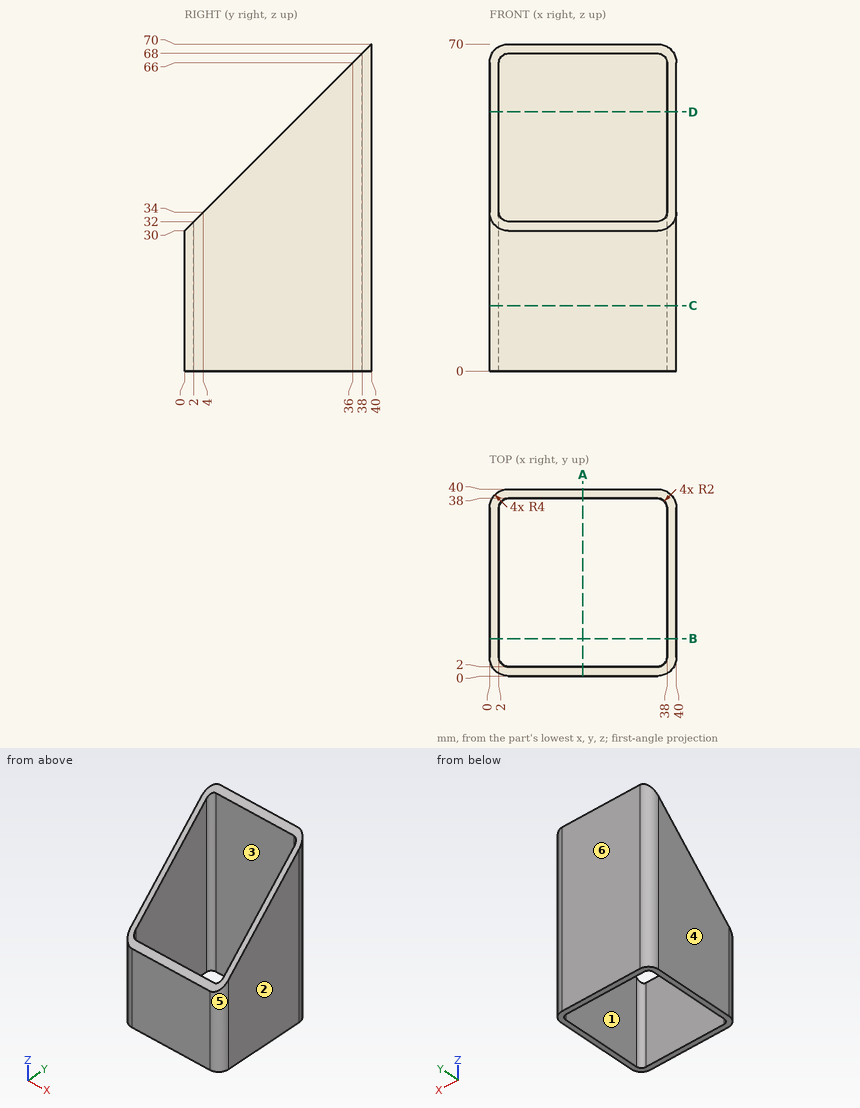
Job drawing, mm, ordinate dimensions from the low corner. One solid piece. A direction names the side the tool comes from. Give positions to 0.01 mm unless a question says otherwise; leave off trailing zeros. Order: outer loops, then holes, each group sorted by start corner. A loop starts at its lowest first (then second) coordinate and runs counter-clockwise, first axis right, second up. Notation, with made-up numbers: (0.25, 52) - (58.25, 52) arc R16 ccw to (58.25, 66) - close; hole circle Ø10 at (50.5, 66.25). An arc over 180 degrees is marked (long way). Return JSON: item names as keys, results as strings.
1) Cut at C-C, the plane z = 14. Give the cut face in (x, y), plus the area to 3 significant figures.
Geometry says:
{"outline": "(0, 4) arc R4 ccw to (4, 0) - (36, 0) arc R4 ccw to (40, 4) - (40, 36) arc R4 ccw to (36, 40) - (4, 40) arc R4 ccw to (0, 36) - close; hole (2, 4) arc R2 ccw to (4, 2) - (36, 2) arc R2 ccw to (38, 4) - (38, 36) arc R2 ccw to (36, 38) - (4, 38) arc R2 ccw to (2, 36) - close", "area": "294 mm²"}
2) 3-axis set-ups, long thin cutter, end or side, ignore diameter. For the marked faces 1 and 2: which of +Z, -Z, +X, -X, +Y, -Y reach the whole face in a straight line?
Geometry says:
{"face 1": "+Z, -Z", "face 2": "+Z, -Z, +X, +Y, -Y"}
3) Pull direction Y, two halves, no side cores. Call the marked faces 3, 4, 5 and 6: pulls with the +Y half, pulls with the -Y half, needs draft (parallel to the pull), parting line crosses it, or undercut.
Geometry says:
{"face 3": "undercut", "face 4": "needs draft", "face 5": "pulls with the -Y half", "face 6": "pulls with the +Y half"}
4) Cut at D-D, the plane z = 55.5. Give the cut face in (x, y), plus the area to 3 significant figures.
Geometry says:
{"outline": "(0, 25.5) - (2, 25.5) - (2, 36) arc R2 cw to (4, 38) - (36, 38) arc R2 cw to (38, 36) - (38, 25.5) - (40, 25.5) - (40, 36) arc R4 ccw to (36, 40) - (4, 40) arc R4 ccw to (0, 36) - close", "area": "125 mm²"}
5) Probe line 1 (X direction, y = 11, z = 36.5); line 2 (Y direction, x = 26, z = 53). List the from-to ranges inside material, lowest first. Write a range as from..to.
Geometry says:
{"line 1": "0..2, 38..40", "line 2": "38..40"}
6) Cut at A-A, the plane x = 20. Give the cut face in (y, z), plus the area to 3 significant figures.
Geometry says:
{"outline": "(0, 0) - (2, 0) - (2, 32) - (0, 30) - close; (38, 0) - (40, 0) - (40, 70) - (38, 68) - close", "area": "200 mm²"}
7) Flat gauge pin, fed straight in: P1, Ø3, axis at x = 15, z = 13, coming from the -Y side. Where does the tip first touch, or does it go through?
Geometry says:
{"P1": "y = 0"}
8) Cut at B-B, the plane y = 8. Give the cut face in (x, z).
Geometry says:
{"outline": "(0, 0) - (2, 0) - (2, 38) - (0, 38) - close; (38, 0) - (40, 0) - (40, 38) - (38, 38) - close"}
